Can you work these out from the model? Positions are in its coordinate system, mm. A direction names the side the tool comes from. Coordinates: 2 decimals unless noted, no trailing zeros. Write each loop counter-clockwise with the first axis right and the second up, starting at its lowest first coordinate (ties: lowest second). Pieces come first, ordered by that corner, then holes. Notation, with made-up numbers: (2, 9.5) - (21, 9.5) arc R20 ccw to (21, 32.5) - close; hole circle Ø1 at (41, 78.25). An arc over 180 degrees is marked (long way). Write each question's results on one line, items separated by ' | '. Start each with the question number.
Autodesk Inventor part; units mm, degrees
ref_plane "YZ Plane" through (0, 0, 0) normal (1, 0, 0) x (0, 1, 0)
ref_plane "XZ Plane" through (0, 0, 0) normal (0, 1, 0) x (-1, 0, 0)
ref_plane "XY Plane" through (0, 0, 0) normal (0, 0, 1) x (1, 0, 0)
sketch "Sketch1" plane through (0, 0, 0) normal (0, 1, 0) x (-1, 0, 0)
  line L0 (0, 0) -> (-4.064, 0)
  line L1 (-4.064, 0) -> (-4.064, -9.398)
  line L2 (-4.064, -9.398) -> (0, -9.398)
  line L3 (0, -9.398) -> (0, 0)
  dimension "d0" = 4.064
  dimension "d1" = 9.398
extrude "Extrusion1" add sketch "Sketch1" along normal blind 20.32
sketch "Sketch3" plane through (4.064, 0, 0) normal (1, 0, 0) x (0, 0, -1)
  line L0 (9.398, 20.32) -> (0, 20.32)
  line L1 (9.398, 0) -> (9.398, 20.32)
  line L2 (0, 20.32) -> (9.398, 20.32)
  line L3 (9.398, 20.32) -> (9.398, 15.494)
  line L4 (9.398, 15.494) -> (0, 15.494)
  line L5 (0, 15.494) -> (0, 20.32)
  point P0 (0, 0)
  dimension "d5" = 4.826
extrude "Extrusion2" add sketch "Sketch3" along normal blind 5.588
sketch "Sketch4" plane through (4.064, 15.494, -9.398) normal (0, -1, 0) x (1, 0, 0)
  line L0 (5.588, 0) -> (5.588, 9.398)
  line L1 (-4.064, 0) -> (5.588, 0)
  line L2 (5.588, 9.398) -> (3.048, 9.398)
  line L3 (3.048, 9.398) -> (3.048, 0)
  line L4 (3.048, 0) -> (5.588, 0)
  line L5 (5.588, 0) -> (5.588, 9.398)
  point P0 (-4.064, 9.398)
  dimension "d8" = 2.54
extrude "Extrusion3" add sketch "Sketch4" along normal blind 12.7
properties part number "Mount Male"
Q1. If we section it at B-B (z = -3.75): Please give me the cut outline in (x, y), then the cut area to 3 significant figures.
Q2. I'm going to push flat-ended pins straight in: pin 1 Ø3.5 at (x, z) = (5, -5) entering from -Y; pin 2 Ø3 at (x, z) = (9, -4.5) entering from -Y. Where does each tip first touch, or does it pass through?
Q3. If we section it at C-C (x = 7.5): Please give me the cut outline in (y, z), then the cut area to 3 significant figures.
Q4. I need wall thicknesses on line 1 along X through (y, z) = (7, -1.75); line 2 along Y through (x, z) = (9, -6.5); line 3 along X through (y, z) = (2.25, -3.75). Which ranges of each line are inside material? Lowest first, please. Write a range as from..to.
Q5. If we section it at A-A (y = 5): Please give me the cut outline in (x, z), then the cut area to 3 significant figures.
Q6. For faces 4 (the face through (8, 2.794, -5)), 5 (the face through (6, 15.494, -5)), 6 (the face through (3.7, 12.6, -9.398)), which set-ups out of +Z, -Z, +X, -X, +Y, -Y let a thin tool reach every point of the face, with its end or its side?
Q7. Thinking about a two-plate mould opening in X: for faces 1 (the face through (2, 0, -5)), 2 (the face through (0, 10, -5)), 3 (the face through (4.064, 8, -5)), which applies, pulls with the +X half, pulls with the -X half, needs draft (parallel to the pull), parting line crosses it, or undercut?
Answer list:
1) outline: (0, 0) - (4.06, 0) - (4.06, 15.49) - (7.11, 15.49) - (7.11, 2.79) - (9.65, 2.79) - (9.65, 20.32) - (0, 20.32) - close | area: 142 mm2
2) pin 1: stops at y = 0 | pin 2: stops at y = 2.79
3) outline: (2.79, -9.4) - (20.32, -9.4) - (20.32, 0) - (2.79, 0) - close | area: 165 mm2
4) line 1: x = 0..4.06, 7.11..9.65 | line 2: y = 2.79..20.32 | line 3: x = 0..4.06
5) outline: (0, -9.4) - (4.06, -9.4) - (4.06, 0) - (0, 0) - close; (7.11, -9.4) - (9.65, -9.4) - (9.65, 0) - (7.11, 0) - close | area: 62.1 mm2
6) face 4: +Z, -Z, +X, -Y | face 5: +Z, -Z, -Y | face 6: -Z, +X, -X, +Y, -Y
7) face 1: needs draft | face 2: pulls with the -X half | face 3: undercut
